from build123d import *

# Parameters (mm, degrees)
F0_R     = 21.275
F0_R_2   = 17.775
F1_DEPTH = 17
F2_R     = 31.5
F2_R_2   = 17.775
F3_DEPTH = 2.5
F4_SIZE2 = 2.9
F4_SIZE  = 1
F5_SIZE  = 0.5
F6_SIZE  = 1


with BuildPart() as f1:
    # F0 (on Top) → F1 (new body)
    with BuildSketch(Plane.XY):
        Circle(F0_R)
        Circle(F0_R_2, mode=Mode.SUBTRACT)
    extrude(amount=F1_DEPTH)

    # F2 (on face) → F3 (join)
    with BuildSketch(Plane.XY.offset(17)):
        Circle(F2_R)
        Circle(F2_R_2, mode=Mode.SUBTRACT)
    extrude(amount=F3_DEPTH)

    # F4
    f4_edges = [f1.edges().sort_by_distance(p)[0] for p in [
        (-31.5, 0, 17),
    ]]
    f4_side = f1.faces().sort_by_distance((-31.5, 0, 18.25))[0]
    chamfer(f4_edges, length=F4_SIZE, length2=F4_SIZE2, reference=f4_side)

    # F5
    f5_edges = [f1.edges().sort_by_distance(p)[0] for p in [
        (-21.275, 0, 0),
    ]]
    chamfer(f5_edges, length=F5_SIZE)

    # F6
    f6_edges = [f1.edges().sort_by_distance(p)[0] for p in [
        (-17.775, 0, 19.5),
    ]]
    chamfer(f6_edges, length=F6_SIZE)


solid = f1.part
Geometry: final body of the model. Coordinates: model frame, mm. A direction names the side the tool comes from. Coordinates: 2 decimals unless noted, no trailing zeros. Loops run counter-clockwise (first coordinate to the right, second up) from the corner with the lowest first, then second, coordinate; pieces in that order, holes last. Notation, with made-up numbers: (51, 22) - (102, 22) arc R31 ccw to (102, 49) - close; hole circle Ø10 at (35.25, -9.75). An arc over 180 degrees is marked (long way). Put each result on its own line as item: value. Start each with the question number.
Q1. Pin query (flat end, axial travel): pin 1 Ø8 at (x, z) = (22.5, 16.5) entering from -Y; pin 2 Ø2 at (y, z) = (-7, 2) entering from -X; pin 3 Ø5 at (x, z) = (-24, 4.5) entering from -Y; pin 4 Ø1 at (x, z) = (0.5, 3) entering from -Y (3 decimals). Return the tip coordinate at first contact, or that it passes through.
Q2. Cut plane C-C, the plane z = 2.5. Return loops of the section in (x, y) (3 decimals).
Q3. Cut plane A-A, the plane y = 0. Return loops of the section in (x, z) (3 decimals).
Q4. Line query: line 1 (Y direction, x = 0, z = 5.5) (3 decimals); line 2 (Z direction, x = 19.5, y = -10); line 3 (X direction, y = 13.5, z = 4). Output: solid intervals per line, ascending.
Q5. Pull-direction query (Y, two-part tool) for faces 1 (the cylindrical face through (-3.853, -17.352, 9.12)), 2 (the cylindrical face through (-4.101, 31.232, 18.74)), 3 (the flat face through (14, -14, 19.5)); classes: released by +Y, released by -Y, zero draft, split by the parting line, or undercut.
Q6. Set-up query: faces 4 (the flat face through (17, 6, 0)), 5 (the cylindrical face through (-16.88, -12.95, 8.63)). Return all of +Z, -Z, +X, -X, +Y, -Y with unobstructed straight access to the full face (end or side cutting, diameter ignored); none if empty.
Filled sheet:
1. pin 1: y = -25.28
1. pin 2: x = -20.41
1. pin 3: through
1. pin 4: y = -21.275
2. outline: circle Ø42.55 at (0, 0); hole circle Ø35.55 at (0, 0)
3. outline: (-31.5, 18) - (-28.6, 17) - (-21.275, 17) - (-21.275, 0.5) - (-20.775, 0) - (-17.775, 0) - (-17.775, 18.5) - (-18.775, 19.5) - (-31.5, 19.5) - close; (17.775, 0) - (20.775, 0) - (21.275, 0.5) - (21.275, 17) - (28.6, 17) - (31.5, 18) - (31.5, 19.5) - (18.775, 19.5) - (17.775, 18.5) - close
4. line 1: -21.275 to -17.775, 17.775 to 21.275
4. line 2: 17 to 19.5
4. line 3: -16.44 to -11.56, 11.56 to 16.44
5. face 1: undercut
5. face 2: split by the parting line
5. face 3: zero draft
6. face 4: -Z, +X, -X, +Y, -Y
6. face 5: -Z
